Can you work these out from the model? Positions are in its coordinate system, mm. A direction names the side the tool comes from. Give positions to 0.01 mm unless a question says otherwise; leave off trailing zeros. Order: outer loops, then holes, each group sorted by start corner. A loop starts at its lowest first (then second) coordinate and runs counter-clockwise, first axis right, second up. Notation, with made-up numbers: (16, 23.5) - (46, 23.5) arc R31 cw to (46, 60.5) - close; hole circle Ø11 at (11, -18). An arc over 180 degrees is marked (long way). Answer as CSV lines item,"result".
```python
from build123d import *

# Parameters (mm, degrees)
EXTRUDE_565_DEPTH = 18.7
SKETCH_2_R        = 15
EXTRUDE_1_DEPTH   = 70
CHAMFER_1_SIZE    = 3.5


with BuildPart() as part:
    # Эскиз1 → Extrude 565 (new body)
    with BuildSketch(Plane(origin=(0, 0, 0), x_dir=(0, 0, -1), z_dir=(1, 0, 0))):
        Polygon((26.558112383, 0), (13.279056191, 23), (-13.279056191, 23), (-26.558112383, 0), (-13.279056191, -23), (13.279056191, -23), align=None)
    extrude(amount=EXTRUDE_565_DEPTH)

    # Эскиз2 → Бобышка-Вытянуть1 (add)
    with BuildSketch(Plane.ZY):
        Circle(SKETCH_2_R)
    extrude(amount=EXTRUDE_1_DEPTH)

    # Фаска1
    chamfer_1_edges = [part.edges().sort_by_distance(p)[0] for p in [
        (-70, 0, -15),
    ]]
    chamfer(chamfer_1_edges, length=CHAMFER_1_SIZE)

    # Эскиз3 (on Front Plane) → Вырез-Вращением1 (revolve, cut)
    with BuildSketch(Plane.XY, mode=Mode.PRIVATE) as cut_revolve_1_sk:
        Polygon((18.7, 26.558112383), (18.7, 21.85), (15.981770048, 26.558112383), align=None)
    revolve(cut_revolve_1_sk.sketch.rotate(Axis((22, 0, 0), (-1, 0, 0)), 90), axis=Axis((22, 0, 0), (-1, 0, 0)), mode=Mode.SUBTRACT)


solid = part.part
```
1) I want a section at C-C on x = -30. Write out the boundary of the cut face in (y, z).
Answer block:
outline,"circle Ø30 at (0, 0)"
2) I want a section at A-A on z = 0. Write out the boundary of the cut face in (x, y).
Answer block:
outline,"(-70, -11.5) - (-66.5, -15) - (0, -15) - (0, -23) - (18.04, -23) - (18.7, -21.85) - (18.7, 21.85) - (18.04, 23) - (0, 23) - (0, 15) - (-66.5, 15) - (-70, 11.5) - close"
3) Which directions (+Z, -Z, +X, -X, +Y, -Y) give clear straight access to the entire face, cutting with the end or side of a thin tool? Please do faces 1 (the flat face through (8.892, 11.661, 19.826)), 2 (the flat face through (0, 11, -11)).
Answer block:
face 1,"+Z, +X, -X, +Y"
face 2,"-X"
4) I'm going to push flat-ended pins straight in: P1, Ø4, axis at x = -23.5, y = -9.5, coming from the +Z side; P2, Ø6, axis at x = -22.5, y = -14, coming from the -Z side; P3, Ø1.5, axis at x = -30, y = 2, coming from the +Z side. Where does each tip first touch, or does it pass through?
Answer block:
P1,"z = 12.99"
P2,"z = -10.2"
P3,"z = 14.95"
5) I need wall thicknesses on line 1 along X through (y, z) = (-2, 21); line 2 along X through (y, z) = (-16, -16.5); line 3 along Z through (x, y) = (-46, -2). Which ranges of each line are inside material? Lowest first, please. Write a range as [from, to].
Answer block:
line 1,"[0, 18.7]"
line 2,"[0, 18.05]"
line 3,"[-14.87, 14.87]"
6) I want a section at B-B on x = 13. Write out the boundary of the cut face in (y, z).
Answer block:
outline,"(-23, -13.28) - (0, -26.56) - (23, -13.28) - (23, 13.28) - (0, 26.56) - (-23, 13.28) - close"
